Work out the finished part from the listing and answer in its coordinate system (mm). A direction names the side the tool comes from. Coordinates: 2 decimals unless noted, no trailing zeros. Write each loop counter-clockwise with the first axis right and the second up, starting at its lowest first coordinate (ties: lowest second). Pieces come first, ordered by that corner, then holes. Notation, with made-up numbers: (-35.75, -1) -> (13.25, -1) arc R29 cw to (13.25, 31) -> close; hole circle Ø10 at (-32, 41). An arc over 180 degrees is marked (long way). Write each question's results on one line, items separated by ' | '. Start each with the question number.
from build123d import *

# Parameters (mm, degrees)
F0_W          = 12.7
F0_H          = 25.4
F0_H_2        = 50.8
F0_H_3        = 88.9
F0_H_4        = 101.6
F1_DEPTH      = 152.4
F2_R          = 25.532371
F3_DEPTH      = 81.28
F3_DEPTH_BACK = 83.82


with BuildPart() as f1:
    # F0 (on Right) → F1 (new body)
    with BuildSketch(Plane.YZ):
        Polygon((-68.94286, 0), (-81.64286, 0), (-81.64286, -12.7), (83.45714, -12.7), (83.45714, 0), (70.75714, 0), (32.65714, 0), (19.95714, 0), (-18.14286, 0), (-30.84286, 0), align=None)
        with Locations((77.10714, 12.7)):
            Rectangle(F0_W, F0_H)
        with Locations((26.30714, 25.4)):
            Rectangle(F0_W, F0_H_2)
        with Locations((-24.49286, 44.45)):
            Rectangle(F0_W, F0_H_3)
        with Locations((-75.29286, 50.8)):
            Rectangle(F0_W, F0_H_4)
    extrude(amount=F1_DEPTH)

    # F2 (on Front) → F3 (join, two sides)
    with BuildSketch(Plane.XZ) as f3_sk:
        with Locations((76.2, 44.45)):
            Circle(F2_R)
    extrude(amount=F3_DEPTH)
    extrude(f3_sk.sketch, amount=-F3_DEPTH_BACK)


solid = f1.part
1. Find section D-D on z = 44.45. Give the vertices of the cut face in (x, y).
2. Find the intervals of material crossed by L1, parallel to Y at x = 19.5, z = 34; L2, parallel to Y at x = 116, z = 3; L3, parallel to Z at x = 119.5, y = -63.5, in increasing order.
3. Find section A-A on z = 11. Give the vertices of the cut face in (x, y).
4. Determine the mould class of faces 1 (the face through (75, -25, 88.9)), 2 (the face through (76, 83.82, 45)), 3 (the face through (75, 32.657, 14)) for opening direction Y: pulls with the +Y half, pulls with the -Y half, needs draft (parallel to the pull), parting line crosses it, or undercut.
5. For faces 4 (the face through (89.926, -49.626, 65.979)), 5 (the face through (25, 26, 50.8)), 6 (the face through (152.4, -24, 24)), 7 (the face through (75, 52, 0)), 8 (the face through (126, 26, 50.8)), determine the directions among +Z, -Z, +X, -X, +Y, -Y from which every point of the face is accessible in a straight line to the end or side of a thin tool.
6. Given pin 1 Ø11.5 at (x, z) = (96.5, 11) entering from +Y; pin 2 Ø6.5 at (x, y) = (30, 77) entering from +Z; pin 3 Ø4 at (x, y) = (41.5, -27.5) entering from +Z, each flat-ended and moving along its own axis, determine where each tip first touches the part or whether it passes through.
7. Find section B-B on y = 40. Give the vertices of the cut face in (x, z), and give its area (3 significant figures).
8. Find section C-C on x = 76.2. Give the vertices of the cut face in (y, z).
Ans:
1) outline: (0, -81.64) -> (152.4, -81.64) -> (152.4, -68.94) -> (101.73, -68.94) -> (101.73, -30.84) -> (152.4, -30.84) -> (152.4, -18.14) -> (101.73, -18.14) -> (101.73, 19.96) -> (152.4, 19.96) -> (152.4, 32.66) -> (101.73, 32.66) -> (101.73, 83.82) -> (50.67, 83.82) -> (50.67, 32.66) -> (0, 32.66) -> (0, 19.96) -> (50.67, 19.96) -> (50.67, -18.14) -> (0, -18.14) -> (0, -30.84) -> (50.67, -30.84) -> (50.67, -68.94) -> (0, -68.94) -> close
2) L1: y = -81.64 to -68.94, -30.84 to -18.14, 19.96 to 32.66 | L2: y = -81.64 to -68.94, -30.84 to -18.14, 19.96 to 32.66, 70.76 to 83.46 | L3: z = -12.7 to 0
3) outline: (0, -81.64) -> (152.4, -81.64) -> (152.4, -68.94) -> (0, -68.94) -> close; (0, -30.84) -> (152.4, -30.84) -> (152.4, -18.14) -> (0, -18.14) -> close; (0, 19.96) -> (152.4, 19.96) -> (152.4, 32.66) -> (0, 32.66) -> close; (0, 70.76) -> (152.4, 70.76) -> (152.4, 83.46) -> (0, 83.46) -> close
4) face 1: needs draft | face 2: pulls with the +Y half | face 3: undercut
5) face 4: none | face 5: +Z, -X, +Y | face 6: +Z, -Z, +X, +Y, -Y | face 7: +X, -X | face 8: +Z, +X, +Y
6) pin 1: stops at y = 83.46 | pin 2: stops at z = 25.4 | pin 3: stops at z = 88.9
7) outline: (0, -12.7) -> (152.4, -12.7) -> (152.4, 0) -> (0, 0) -> close; circle Ø51.06 at (76.2, 44.45) | area: 3,980 mm²
8) outline: (-81.64, -12.7) -> (83.46, -12.7) -> (83.46, 18.92) -> (83.82, 18.92) -> (83.82, 69.98) -> (-18.14, 69.98) -> (-18.14, 88.9) -> (-30.84, 88.9) -> (-30.84, 69.98) -> (-68.94, 69.98) -> (-68.94, 101.6) -> (-81.64, 101.6) -> close; hole (-68.94, 0) -> (-30.84, 0) -> (-30.84, 18.92) -> (-68.94, 18.92) -> close; hole (-18.14, 0) -> (19.96, 0) -> (19.96, 18.92) -> (-18.14, 18.92) -> close; hole (32.66, 0) -> (70.76, 0) -> (70.76, 18.92) -> (32.66, 18.92) -> close
